For this review, take the finished solid that the model builds, in its own axes (mm). A direction names the side the tool comes from. Give positions to 0.01 mm unless a question says otherwise; leave off trailing zeros. Order: outer loops, then holes, each group sorted by start corner. A loop starts at its lowest first (then second) coordinate and runs counter-clockwise, first axis right, second up. Notation, with made-up numbers: (31.5, 23) -> (43.5, 23) arc R25 ccw to (43.5, 38) -> close; hole circle Ø4 at (17, 53.5). An arc over 180 degrees is marked (long way). Return JSON: item names as keys, results as strings. Group by question number.
1) Add section A-A (y = -8.5). Give the boundary of the cut face in (x, z), then the cut area to 3 significant figures.
2) Add section B-B (x = -46). Give the boundary of the cut face in (y, z), then the cut area to 3 significant figures.
3) The part is to be moulded in two halves that separate along X. For faces 1 (the face through (-13.2, -47, 1.5)), 2 (the face through (8, -1, 4)), 3 (the face through (-73.57, 45.5, 1.49)), say which applies: released by +X, released by -X, zero draft, split by the parting line, or undercut.
4) Add section C-C (y = 32). Give the boundary of the cut face in (x, z).
5) For faces 4 (the face through (31, -1, 4)), 5 (the face through (60.6, -28.8, 6)), 6 (the face through (32, -1, 4)), list the 3-axis set-ups (+Z, -Z, +X, -X, +Y, -Y) from which the entire face can be reached by the end or side of a thin tool; tool diameter is ignored.
6) Insertion check: P1, Ø1.8, axis at x = 75, y = 42, coming from the +Z side; P2, Ø1.1, axis at x = 42.5, y = -23, coming from the -Z side; P3, Ø0.8, axis at x = 0.5, z = 5, coming from the -Y side; P4, Ø12, axis at x = -30.5, y = -11, coming from the +Z side. Each pin has a flat end and moves straight along its axis. Give the tip position at first contact, or say it passes through.
7) To check wall thickness, follow line 1 along X through (y, z) = (-29, 1.75); line 2 along X through (y, z) = (0, 1.45); line 3 along X through (y, z) = (-29, 5). State the ranges of each line that lie inside material, in increasing order.
from build123d import *

# Parameters (mm, degrees)
BOSS_EXTRUDE1_DEPTH                           = 2
CSK_FOR_0_FLAT_HEAD_MACHINE_SCREW1_AT_2_COUNT = 2
CSK_FOR_0_FLAT_HEAD_MACHINE_SCREW1_AT_2_PITCH = 42
CSK_FOR_0_FLAT_HEAD_MACHINE_SCREW1_AT_3_COUNT = 2
CSK_FOR_0_FLAT_HEAD_MACHINE_SCREW1_AT_3_PITCH = 84
CSK_FOR_0_FLAT_HEAD_MACHINE_SCREW1_AT_4_COUNT = 2
CSK_FOR_0_FLAT_HEAD_MACHINE_SCREW1_AT_4_PITCH = 112.609946275
CSK_FOR_0_FLAT_HEAD_MACHINE_SCREW1_AT_5_COUNT = 2
CSK_FOR_0_FLAT_HEAD_MACHINE_SCREW1_AT_5_PITCH = 167.573864311
CSK_FOR_0_FLAT_HEAD_MACHINE_SCREW1_AT_6_COUNT = 2
CSK_FOR_0_FLAT_HEAD_MACHINE_SCREW1_AT_6_PITCH = 150.960259671
CSK_FOR_0_FLAT_HEAD_MACHINE_SCREW1_AT_7_COUNT = 2
CSK_FOR_0_FLAT_HEAD_MACHINE_SCREW1_AT_7_PITCH = 145
CSK_FOR_0_FLAT_HEAD_MACHINE_SCREW1_AT_8_COUNT = 2
CSK_FOR_0_FLAT_HEAD_MACHINE_SCREW1_AT_8_PITCH = 75
FILLET1_R                                     = 1
SKETCH9_W                                     = 22
SKETCH9_H                                     = 76
CUT_EXTRUDE2_DEPTH                            = 1
SKETCH9_5_W                                   = 24
SKETCH9_5_H                                   = 78
SKETCH9_5_W_2                                 = 22
SKETCH9_5_H_2                                 = 76
BOSS_EXTRUDE4_DEPTH                           = 5
SKETCH11_W                                    = 4
SKETCH11_H                                    = 2
CUT_EXTRUDE4_DEPTH                            = 5
SKETCH13_W                                    = 4
SKETCH13_H                                    = 2
CUT_EXTRUDE5_DEPTH                            = 1
SKETCH14_W                                    = 4
SKETCH14_H                                    = 1
CUT_EXTRUDE6_DEPTH                            = 1
SKETCH15_W                                    = 4
SKETCH15_H                                    = 1
CUT_EXTRUDE7_DEPTH                            = 1
BOSS_EXTRUDE5_DEPTH                           = 4
SKETCH9_8_W                                   = 17
SKETCH9_8_H                                   = 27
CUT_EXTRUDE10_DEPTH                           = 1
SKETCH17_W                                    = 2
SKETCH17_H                                    = 2
CUT_EXTRUDE11_DEPTH                           = 1
SKETCH18_W                                    = 2
SKETCH18_H                                    = 2
CUT_EXTRUDE12_DEPTH                           = 21
CUT_EXTRUDE12_DEPTH_BACK                      = 1
CUT_EXTRUDE13_DEPTH                           = 1
BOSS_EXTRUDE6_DEPTH                           = 4


with BuildPart() as part:
    # Sketch1 → Boss-Extrude1 (new body)
    with BuildSketch(Plane.XY):
        with BuildLine():
            Line((-70, 47), (75, 47))
            ThreePointArc((75, 47), (78.535533906, 45.535533906), (80, 42))
            Line((80, 42), (80, -42))
            ThreePointArc((80, -42), (78.535533906, -45.535533906), (75, -47))
            Line((75, -47), (-70, -47))
            ThreePointArc((-70, -47), (-73.535533906, -45.535533906), (-75, -42))
            Line((-75, -42), (-75, 42))
            ThreePointArc((-75, 42), (-73.535533906, 45.535533906), (-70, 47))
        make_face()
    extrude(amount=BOSS_EXTRUDE1_DEPTH)

    # Sketch8 → CSK for _0 Flat Head Machine Screw1 (revolve, cut)
    with BuildSketch(Plane(origin=(75, 42, 0), x_dir=(0, 1, 0), z_dir=(1, 0, 0))):
        Polygon((0, 0), (0, 2), (1.500000048, 2), (1.500000048, 0.575184076), (1.999999937, 0), align=None)
    csk_for_0_flat_head_machine_screw1 = revolve(axis=Axis((75, 42, -6.35), (0, 0, 1)), mode=Mode.SUBTRACT)

    # CSK for _0 Flat Head Machine Screw1 at 2: CSK for _0 Flat Head Machine Screw1 ×2
    with Locations(*[(0, -i * CSK_FOR_0_FLAT_HEAD_MACHINE_SCREW1_AT_2_PITCH, 0) for i in range(1, CSK_FOR_0_FLAT_HEAD_MACHINE_SCREW1_AT_2_COUNT)]):
        add(csk_for_0_flat_head_machine_screw1, mode=Mode.SUBTRACT)

    # CSK for _0 Flat Head Machine Screw1 at 3: CSK for _0 Flat Head Machine Screw1 ×2
    with Locations(*[(0, -i * CSK_FOR_0_FLAT_HEAD_MACHINE_SCREW1_AT_3_PITCH, 0) for i in range(1, CSK_FOR_0_FLAT_HEAD_MACHINE_SCREW1_AT_3_COUNT)]):
        add(csk_for_0_flat_head_machine_screw1, mode=Mode.SUBTRACT)

    # CSK for _0 Flat Head Machine Screw1 at 4: CSK for _0 Flat Head Machine Screw1 ×2
    with Locations(*[Vector(-0.666015769, -0.745937662, 0) * (i * CSK_FOR_0_FLAT_HEAD_MACHINE_SCREW1_AT_4_PITCH) for i in range(1, CSK_FOR_0_FLAT_HEAD_MACHINE_SCREW1_AT_4_COUNT)]):
        add(csk_for_0_flat_head_machine_screw1, mode=Mode.SUBTRACT)

    # CSK for _0 Flat Head Machine Screw1 at 5: CSK for _0 Flat Head Machine Screw1 ×2
    with Locations(*[Vector(-0.865290065, -0.501271486, 0) * (i * CSK_FOR_0_FLAT_HEAD_MACHINE_SCREW1_AT_5_PITCH) for i in range(1, CSK_FOR_0_FLAT_HEAD_MACHINE_SCREW1_AT_5_COUNT)]):
        add(csk_for_0_flat_head_machine_screw1, mode=Mode.SUBTRACT)

    # CSK for _0 Flat Head Machine Screw1 at 6: CSK for _0 Flat Head Machine Screw1 ×2
    with Locations(*[Vector(-0.960517691, -0.278218917, 0) * (i * CSK_FOR_0_FLAT_HEAD_MACHINE_SCREW1_AT_6_PITCH) for i in range(1, CSK_FOR_0_FLAT_HEAD_MACHINE_SCREW1_AT_6_COUNT)]):
        add(csk_for_0_flat_head_machine_screw1, mode=Mode.SUBTRACT)

    # CSK for _0 Flat Head Machine Screw1 at 7: CSK for _0 Flat Head Machine Screw1 ×2
    with Locations(*[(-i * CSK_FOR_0_FLAT_HEAD_MACHINE_SCREW1_AT_7_PITCH, 0, 0) for i in range(1, CSK_FOR_0_FLAT_HEAD_MACHINE_SCREW1_AT_7_COUNT)]):
        add(csk_for_0_flat_head_machine_screw1, mode=Mode.SUBTRACT)

    # CSK for _0 Flat Head Machine Screw1 at 8: CSK for _0 Flat Head Machine Screw1 ×2
    with Locations(*[(-i * CSK_FOR_0_FLAT_HEAD_MACHINE_SCREW1_AT_8_PITCH, 0, 0) for i in range(1, CSK_FOR_0_FLAT_HEAD_MACHINE_SCREW1_AT_8_COUNT)]):
        add(csk_for_0_flat_head_machine_screw1, mode=Mode.SUBTRACT)

    # Fillet1
    fillet1_edges = [part.edges().sort_by_distance(p)[0] for p in [
        (-75, 0, 0),
        (-73.535533906, 45.535533906, 0),
        (2.5, 47, 0),
        (78.535533906, 45.535533906, 0),
        (80, 0, 0),
        (78.535533906, -45.535533906, 0),
        (2.5, -47, 0),
        (-73.535533906, -45.535533906, 0),
    ]]
    fillet(fillet1_edges, radius=FILLET1_R)

    # Sketch9 → Cut-Extrude2 (cut)
    with BuildSketch(Plane.XY.offset(2)):
        with Locations((20, 0)):
            Rectangle(SKETCH9_W, SKETCH9_H)
    extrude(amount=-CUT_EXTRUDE2_DEPTH, mode=Mode.SUBTRACT)

    # Sketch9_5 → Boss-Extrude4 (add)
    with BuildSketch(Plane.XY.offset(2)):
        with Locations((20, 0)):
            Rectangle(SKETCH9_5_W, SKETCH9_5_H)
        with Locations((20, 0)):
            Rectangle(SKETCH9_5_W_2, SKETCH9_5_H_2, mode=Mode.SUBTRACT)
    extrude(amount=BOSS_EXTRUDE4_DEPTH)

    # Sketch11 → Cut-Extrude4 (cut)
    with BuildSketch(Plane(origin=(0, 39, 0), x_dir=(1, 0, 0), z_dir=(0, 1, 0))):
        with Locations((13, -3)):
            Rectangle(SKETCH11_W, SKETCH11_H)
    extrude(amount=-CUT_EXTRUDE4_DEPTH, mode=Mode.SUBTRACT)

    # Sketch13 → Cut-Extrude5 (cut)
    with BuildSketch(Plane.XZ.offset(39)):
        with Locations((27, 3)):
            Rectangle(SKETCH13_W, SKETCH13_H)
    extrude(amount=-CUT_EXTRUDE5_DEPTH, mode=Mode.SUBTRACT)

    # Sketch14 → Cut-Extrude6 (cut)
    with BuildSketch(Plane.XZ.offset(-38)):
        with Locations((13, 1.5)):
            Rectangle(SKETCH14_W, SKETCH14_H)
    extrude(amount=-CUT_EXTRUDE6_DEPTH, mode=Mode.SUBTRACT)

    # Sketch15 → Cut-Extrude7 (cut)
    with BuildSketch(Plane(origin=(0, -38, 0), x_dir=(1, 0, 0), z_dir=(0, 1, 0))):
        with Locations((27, -1.5)):
            Rectangle(SKETCH15_W, SKETCH15_H)
    extrude(amount=-CUT_EXTRUDE7_DEPTH, mode=Mode.SUBTRACT)

    # Sketch9_7 → Boss-Extrude5 (add)
    with BuildSketch(Plane.XY.offset(2)):
        Polygon((42, -47), (43, -47), (43, -20), (60, -20), (60, -47), (61, -47), (61, -19), (42, -19), align=None)
    extrude(amount=BOSS_EXTRUDE5_DEPTH)

    # Sketch9_8 → Cut-Extrude10 (cut)
    with BuildSketch(Plane.XY.offset(2)):
        with Locations((51.5, -33.5)):
            Rectangle(SKETCH9_8_W, SKETCH9_8_H)
    extrude(amount=-CUT_EXTRUDE10_DEPTH, mode=Mode.SUBTRACT)

    # Sketch17 → Cut-Extrude11 (cut)
    with BuildSketch(Plane.XZ.offset(20)):
        with Locations((47, 3)):
            Rectangle(SKETCH17_W, SKETCH17_H)
        with Locations((55, 3)):
            Rectangle(SKETCH17_W, SKETCH17_H)
    extrude(amount=-CUT_EXTRUDE11_DEPTH, mode=Mode.SUBTRACT)

    # Sketch18 → Cut-Extrude12 (cut, two sides)
    with BuildSketch(Plane.ZY.offset(-60)) as cut_extrude12_sk:
        with Locations((3, -23)):
            Rectangle(SKETCH18_W, SKETCH18_H)
    extrude(amount=CUT_EXTRUDE12_DEPTH, mode=Mode.SUBTRACT)
    extrude(cut_extrude12_sk.sketch, amount=-CUT_EXTRUDE12_DEPTH_BACK, mode=Mode.SUBTRACT)

    # Sketch19 → Cut-Extrude13 (cut)
    with BuildSketch(Plane.XY.offset(2)):
        with BuildLine():
            Line((30.191318858, -41.849789893), (32, -41.849789893))
            ThreePointArc((32, -41.849789893), (33.414213562, -41.264003455), (34, -39.849789893))
            Line((34, -39.849789893), (34, -16))
            Line((34, -16), (34, 39))
            ThreePointArc((34, 39), (33.414213562, 40.414213562), (32, 41))
            Line((32, 41), (18.235350669, 41))
            Line((18.235350669, 41), (18.235350669, 42))
            Line((18.235350669, 42), (33, 42))
            ThreePointArc((33, 42), (34.414213562, 41.414213562), (35, 40))
            Line((35, 40), (35, -13))
            ThreePointArc((35, -13), (35.585786438, -14.414213562), (37, -15))
            Line((37, -15), (43.101704987, -15))
            Line((43.101704987, -15), (43.101704987, -16))
            Line((43.101704987, -16), (43.101704987, -17))
            Line((43.101704987, -17), (37, -17))
            ThreePointArc((37, -17), (35.585786438, -17.585786438), (35, -19))
            Line((35, -19), (35, -40.849789893))
            ThreePointArc((35, -40.849789893), (34.414213562, -42.264003455), (33, -42.849789893))
            Line((33, -42.849789893), (30.191318858, -42.849789893))
            Line((30.191318858, -42.849789893), (30.191318858, -41.849789893))
        make_face()
    extrude(amount=-CUT_EXTRUDE13_DEPTH, mode=Mode.SUBTRACT)

    # Sketch20 → Boss-Extrude6 (add)
    with BuildSketch(Plane.XY.offset(2)):
        Polygon((0, 0), (0, -23), (1, -23), (1, 1), (-26, 1), (-26, -23), (-25, -23), (-25, 0), align=None)
    extrude(amount=BOSS_EXTRUDE6_DEPTH)


solid = part.part
Evaluation:
{
 "1": {"outline": "(-75, 1) arc R1 ccw to (-74, 0) -> (79, 0) arc R1 ccw to (80, 1) -> (80, 2) -> (35, 2) -> (35, 1) -> (34, 1) -> (34, 2) -> (32, 2) -> (32, 7) -> (31, 7) -> (31, 1) -> (9, 1) -> (9, 7) -> (8, 7) -> (8, 2) -> (1, 2) -> (1, 6) -> (0, 6) -> (0, 2) -> (-25, 2) -> (-25, 6) -> (-26, 6) -> (-26, 2) -> (-75, 2) -> close", "area": "305 mm^2"},
 "2": {"outline": "(-47, 1) arc R1 ccw to (-46, 0) -> (46, 0) arc R1 ccw to (47, 1) -> (47, 2) -> (-47, 2) -> close", "area": "188 mm^2"},
 "3": {"face 1": "zero draft", "face 2": "undercut", "face 3": "released by -X"},
 "4": {"outline": "(-75, 1) arc R1 ccw to (-74, 0) -> (79, 0) arc R1 ccw to (80, 1) -> (80, 2) -> (35, 2) -> (35, 1) -> (34, 1) -> (34, 2) -> (32, 2) -> (32, 7) -> (31, 7) -> (31, 1) -> (9, 1) -> (9, 7) -> (8, 7) -> (8, 2) -> (-75, 2) -> close"},
 "5": {"face 4": "+Z", "face 5": "+Z, +X, +Y, -Y", "face 6": "+Z, +Y, -Y"},
 "6": {"P1": "through", "P2": "z = 0", "P3": "y = -23", "P4": "z = 6"},
 "7": {"line 1": "-75 to 9, 31 to 34, 35 to 43, 60 to 80", "line 2": "-75 to -71.5, -68.5 to 9, 31 to 34, 35 to 73.5, 76.5 to 80", "line 3": "8 to 9, 31 to 32, 42 to 43, 60 to 61"}
}
